For this review, take the finished solid that the model builds, in its own axes (mm). Face numbers are marked on the shaded views. Coordinates: 2 decimals unless noted, no trailing zeros. Order: outer loops, then holes, each group sorted by start corner. A loop starts at its lowest first (then second) coordinate and runs counter-clockwise, first axis right, second up.
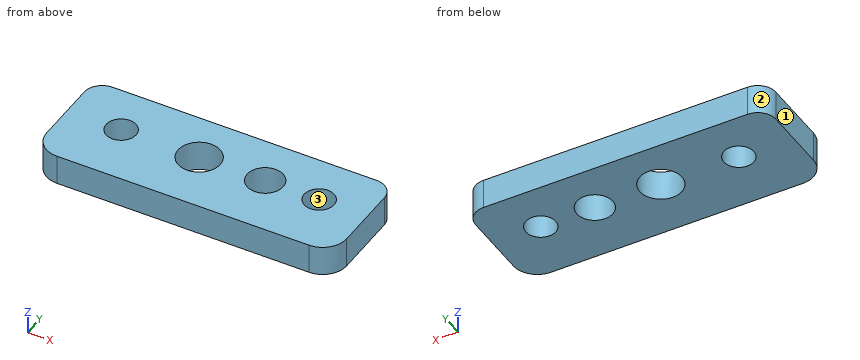
from build123d import *

# Parameters (mm, degrees)
CROQUIS1_W              = 250
CROQUIS1_H              = 90
CROQUIS1_R              = 12.5
CROQUIS1_R_2            = 17.5
CROQUIS1_R_3            = 15
SALIENTE_EXTRUIR1_DEPTH = 25
REDONDEO1_R             = 15
REDONDEO2_R             = 20


with BuildPart() as part:
    # Croquis1 → Saliente-Extruir1 (new body)
    with BuildSketch(Plane.XY):
        with Locations((125, -45)):
            Rectangle(CROQUIS1_W, CROQUIS1_H)
        with Locations((45, -40)):
            Circle(CROQUIS1_R, mode=Mode.SUBTRACT)
        with Locations((110, -40)):
            Circle(CROQUIS1_R_2, mode=Mode.SUBTRACT)
        with Locations((165, -40)):
            Circle(CROQUIS1_R_3, mode=Mode.SUBTRACT)
        with Locations((210, -40)):
            Circle(CROQUIS1_R, mode=Mode.SUBTRACT)
    extrude(amount=SALIENTE_EXTRUIR1_DEPTH)

    # Redondeo1
    redondeo1_edges = [part.edges().sort_by_distance(p)[0] for p in [
        (0, 0, 12.5),
        (250, 0, 12.5),
    ]]
    fillet(redondeo1_edges, radius=REDONDEO1_R)

    # Redondeo2
    redondeo2_edges = [part.edges().sort_by_distance(p)[0] for p in [
        (250, -90, 12.5),
        (0, -90, 12.5),
    ]]
    fillet(redondeo2_edges, radius=REDONDEO2_R)


solid = part.part
1. Take a section at D-D, the plane y = -49.5. Give the boundary of the cut face in (x, z).
Answer below:
outline: (0, 0) - (36.88, 0) - (36.88, 25) - (0, 25) - close; (53.12, 0) - (95.3, 0) - (95.3, 25) - (53.12, 25) - close; (124.7, 0) - (153.39, 0) - (153.39, 25) - (124.7, 25) - close; (176.61, 0) - (201.88, 0) - (201.88, 25) - (176.61, 25) - close; (218.12, 0) - (250, 0) - (250, 25) - (218.12, 25) - close
2. Take a section at C-C, the plane x = 45. Give the boundary of the cut face in (y, z), plus the area to 4 significant figures.
Answer below:
outline: (-90, 0) - (-52.5, 0) - (-52.5, 25) - (-90, 25) - close; (-27.5, 0) - (0, 0) - (0, 25) - (-27.5, 25) - close
area: 1,625 mm2
3. To check wall thickness, follow L1, parallel to Y at x = 45, z = 19.5; L2, parallel to Y at x = 164, z = 11.75; L3, parallel to X at y = -50, z = 3. State the ranges of each line that lie inside material, in increasing order.
Answer below:
L1: y = -90 to -52.5, -27.5 to 0
L2: y = -90 to -54.97, -25.03 to 0
L3: x = 0 to 37.5, 52.5 to 95.64, 124.36 to 153.82, 176.18 to 202.5, 217.5 to 250
4. Take a section at B-B, the plane y = -40. Give the boundary of the cut face in (x, z).
Answer below:
outline: (0, 0) - (32.5, 0) - (32.5, 25) - (0, 25) - close; (57.5, 0) - (92.5, 0) - (92.5, 25) - (57.5, 25) - close; (127.5, 0) - (150, 0) - (150, 25) - (127.5, 25) - close; (180, 0) - (197.5, 0) - (197.5, 25) - (180, 25) - close; (222.5, 0) - (250, 0) - (250, 25) - (222.5, 25) - close
5. Take a section at A-A, the plane x = 165. Give the boundary of the cut face in (y, z), plus the area to 3 significant figures.
Answer below:
outline: (-90, 0) - (-55, 0) - (-55, 25) - (-90, 25) - close; (-25, 0) - (0, 0) - (0, 25) - (-25, 25) - close
area: 1,500 mm2
6. The part is to be moulded in two halves that separate along Y. For the marked faces 1, 2 and 3, say which applies: +Y half, -Y half, draft (parallel to the pull), parting line (faces both ways), or undercut.
Answer below:
face 1: draft
face 2: +Y half
face 3: undercut
